Work out the finished part from the listing and answer in its coordinate system (mm). A direction names the side the tool comes from. Give positions to 0.01 mm unless a question says otherwise; leave off trailing zeros. Order: outer loops, then holes, each group sorted by start corner. A loop starts at its lowest first (then second) coordinate and runs counter-clockwise, first axis right, second up. Notation, with made-up numbers: M 76.25,51.25 L 116.25,51.25 A13 ccw 116.25,57.25 Z; hole C 27.25,44 d10. An arc over 180 degrees is marked long. One line per item, written item: value.
Autodesk Inventor part; units mm, degrees
ref_plane "YZ Plane" through (0, 0, 0) normal (1, 0, 0) x (0, 1, 0)
ref_plane "XZ Plane" through (0, 0, 0) normal (0, 1, 0) x (-1, 0, 0)
ref_plane "XY Plane" through (0, 0, 0) normal (0, 0, 1) x (1, 0, 0)
sketch "Sketch1" plane through (0, 0, 0) normal (0, 0, 1) x (1, 0, 0)
  line L0 (0, -22.5) -> (560, -22.5)
  line L1 (560, -22.5) -> (560, 22.5)
  line L2 (560, 22.5) -> (0, 22.5)
  line L3 (0, 22.5) -> (0, -22.5)
  line L4 (0, -22.5) -> (560, 22.5) construction
  line L5 (560, -22.5) -> (0, 22.5) construction
  point P0 (0, 0)
  point P1 (0, 0)
  dimension "d154" = 560
  dimension "d155" = 45
extrude "Plate3" add sketch "Sketch1" along normal blind 2
sketch "Sketch7" plane through (0, 20.5, 0) normal (0, 1, 0) x (-1, 0, 0)
  line L0 (-560, 0) -> (0, 0)
  line L1 (0, 0) -> (0, 105)
  line L2 (0, 105) -> (-560, 105)
  line L3 (-560, 105) -> (-560, 0)
edge flange "Flange3" height 105 angle 90 thickness 2 bend radius 2.75 thickness toward (0, 1, 0) relief round relief width 2 relief depth 1 edges at (280, 22.5, 2) wall of the first edge with corners at (560, 20.5, 0) (0, 20.5, 0) (0, 20.5, 105) (560, 20.5, 105)
bend "Bend3"
corner "Corner3"
sketch "Sketch11" plane through (0, 20.5, 105) normal (0, -1, 0) x (1, 0, 0)
  line L0 (0, -100.25) -> (560, -100.25)
  line L1 (560, -100.25) -> (560, 0)
  line L2 (560, 0) -> (0, 0)
  line L3 (0, -100.25) -> (0, 0)
  line L4 (0, 0) -> (-23.7581, 0)
  line L5 (-23.7581, 0) -> (-49.4388, -103)
  line L6 (-49.4388, -103) -> (-1, -103)
  line L7 (-1, -103) -> (-1, -100.25)
  line L8 (-1, -100.25) -> (0, -100.25)
  line L9 (560, -103) -> (0, -103)
  line L10 (-1, -103) -> (-46.6039, -91.6297)
  point P0 (0, -105)
  dimension "d193" = 1
  dimension "d194" = 23.7581
  dimension "d195" = 14
  dimension "d203" = 47
extrude "Extrusion6" add sketch "Sketch11" against normal up to surface (2 mm away) contours L8 L7 L10 L5 L4 L3
sketch "Sketch12" plane through (560, 20.5, 4.75) normal (0, -1, 0) x (1, 0, 0)
  line L0 (-511.4632, 69.8575) -> (-545.4236, 78.3248)
  line L1 (-545.4236, 78.3248) -> (-553.8908, 44.3644)
  line L2 (-553.8908, 44.3644) -> (-519.9305, 35.8972)
  line L3 (-519.9305, 35.8972) -> (-511.4632, 69.8575)
  line L4 (-511.4632, 69.8575) -> (-553.8908, 44.3644) construction
  line L5 (-545.4236, 78.3248) -> (-519.9305, 35.8972) construction
  circle A0 centre (-541.1443, 23.1506) radius 5.05
  circle A1 centre (-492.6686, 72.9011) radius 5.05
  circle A2 centre (-560.5893, 89.8356) radius 5.05
  line L6 (-492.6686, 72.9011) -> (-560.5893, 89.8356) construction
  line L7 (-560.5893, 89.8356) -> (-541.1443, 23.1506) construction
  line L8 (-541.1443, 23.1506) -> (-492.6686, 72.9011) construction
  line L9 (-528.4434, 74.0911) -> (-541.1443, 23.1506) construction
  line L10 (-583.7581, 100.25) -> (-606.6039, 8.6203)
  point P0 (-560, -4.75)
  point P1 (-532.677, 57.111)
  point P2 (-543.753, 12.6876)
  dimension "d206" = 35
  dimension "d207" = 35
  dimension "d208" = 10.1
  dimension "d209" = 70
  dimension "d210" = 60
  dimension "d211" = 25
  dimension "d213" = 12
  dimension "d214" = 60
extrude "Cut1" cut sketch "Sketch12" against normal blind 2
pattern_linear "Rectangular Pattern5" count 4 spacing 160 along (1, 0, 0) of "Cut1"
properties part number "MNT-CDF-501 box" material "Stainless Steel"
(1) Section C-C, the plane y = -8.5 is taken. Give the vertices of the cut face in (x, z).
Findings:
outline: M 0,0 L 560,0 L 560,2 L 0,2 Z
(2) Section B-B, the plane x = 99 is taken. Give the vertices of the cut face in (y, z).
Findings:
outline: M -22.5,0 L 17.75,0 A4.75 ccw 22.5,4.75 L 22.5,105 L 20.5,105 L 20.5,4.75 A2.75 cw 17.75,2 L -22.5,2 Z
(3) Section A-A, the plane z = 64 is taken. Give the vertices of the cut face in (x, y), then the cut area to 3 significant figures.
Findings:
outline: M -33.98,20.5 L 9.82,20.5 L 9.82,22.5 L -33.98,22.5 Z; M 45.89,20.5 L 169.82,20.5 L 169.82,22.5 L 45.89,22.5 Z; M 205.89,20.5 L 329.82,20.5 L 329.82,22.5 L 205.89,22.5 Z; M 365.89,20.5 L 489.82,20.5 L 489.82,22.5 L 365.89,22.5 Z; M 525.89,20.5 L 560,20.5 L 560,22.5 L 525.89,22.5 Z
area: 899 mm^2
(4) Find the intervals of material crossed by probe 1 along Y at (x, z) = (141.5, 22); probe 2 along Z at (x, y) = (54, 7), in increasing order. Write a range as from..to.
Findings:
probe 1: y = 20.5..22.5
probe 2: z = 0..2
(5) Given P1, Ø5, axis at x = 362, z = 48.5, coming from the -Y side; P2, Ø6, axis at x = 387.33, z = 77.65, coming from the +Y side; P3, Ø2.5, axis at y = -0.5, z = 2.5, coming from the -X side, each flat-ended and moving along its own axis, determine where each tip first touches the part or whether it passes through.
Findings:
P1: stops at y = 20.5
P2: passes through
P3: stops at x = 0
(6) Which of the six approach directions +Z, -Z, +X, -X, +Y, -Y give full straight-line access (tool end or side, diameter ignored) to faces 1 (the flat face through (276, -2, 2)), 2 (the cylindrical face through (474.366, 21.486, 94.808))?
Findings:
face 1: +Z, +X, -X, -Y
face 2: +Y, -Y
(7) Determine the mould class of faces 3 (the flat face through (252, 20.5, 54)), 4 (the flat face through (-23.483, 21.486, 7.606)), 5 (the cylindrical face through (63.324, 21.486, 74.578)), 6 (the cylindrical face through (382.286, 21.486, 77.873)) for opening direction X: pulls with the +X half, pulls with the -X half, needs draft (parallel to the pull), parting line crosses it, or undercut.
Findings:
face 3: needs draft
face 4: pulls with the -X half
face 5: undercut
face 6: undercut
